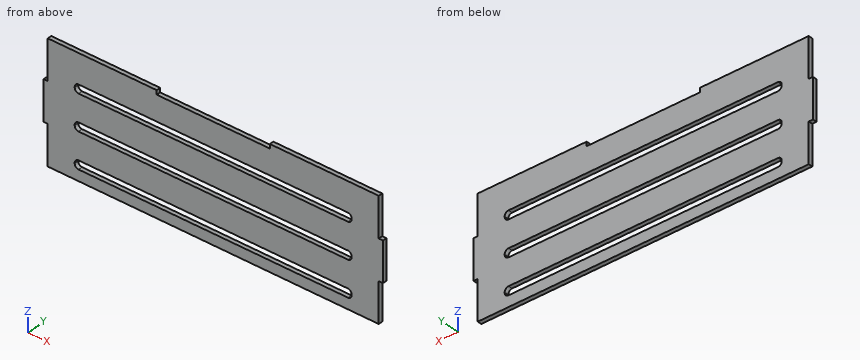
from build123d import *

# Parameters (mm, degrees)
SKETCH1_W           = 490
SKETCH1_H           = 168.89
BOSS_EXTRUDE1_DEPTH = 6
SKETCH2_W           = 163.333333334
SKETCH2_H           = 6
CUT_EXTRUDE1_DEPTH  = 519.324060892
SKETCH4_W           = 6
SKETCH4_H           = 56.296666667
CUT_EXTRUDE3_DEPTH  = 519.324060892
CUT_EXTRUDE4_DEPTH  = 519.324060892
LPATTERN1_COUNT     = 3
LPATTERN1_PITCH     = 50


with BuildPart() as part:
    # Sketch1 → Boss-Extrude1 (new body)
    with BuildSketch(Plane(origin=(0, 0, 0), x_dir=(1, 0, 0), z_dir=(0, 1, 0))):
        with Locations((245, 84.445)):
            Rectangle(SKETCH1_W, SKETCH1_H)
    extrude(amount=BOSS_EXTRUDE1_DEPTH)

    # Sketch2 → Cut-Extrude1 (cut, through all)
    with BuildSketch(Plane(origin=(0, 6, 0), x_dir=(1, 0, 0), z_dir=(0, 1, 0))):
        with Locations((245, 3)):
            Rectangle(SKETCH2_W, SKETCH2_H)
    extrude(amount=-CUT_EXTRUDE1_DEPTH, mode=Mode.SUBTRACT)

    # Sketch4 → Cut-Extrude3 (cut, through all)
    with BuildSketch(Plane(origin=(0, 6, 0), x_dir=(1, 0, 0), z_dir=(0, 1, 0))):
        with Locations((3, 140.741666667)):
            Rectangle(SKETCH4_W, SKETCH4_H)
        with Locations((3, 28.148333334)):
            Rectangle(SKETCH4_W, SKETCH4_H)
        with Locations((487, 28.148333334)):
            Rectangle(SKETCH4_W, SKETCH4_H)
        with Locations((487, 140.741666667)):
            Rectangle(SKETCH4_W, SKETCH4_H)
    extrude(amount=-CUT_EXTRUDE3_DEPTH, mode=Mode.SUBTRACT)

    # Sketch5 → Cut-Extrude4 (cut, through all)
    with BuildSketch(Plane(origin=(0, 6, 0), x_dir=(1, 0, 0), z_dir=(0, 1, 0))):
        with BuildLine():
            Line((50.5, 153.449523313), (439.5, 153.449523313))
            ThreePointArc((439.5, 153.449523313), (443.389087297, 151.838610609), (445, 147.949523313))
            Line((445, 147.949523313), (445, 146.949523313))
            ThreePointArc((445, 146.949523313), (443.389087297, 143.060436016), (439.5, 141.449523313))
            Line((439.5, 141.449523313), (50.5, 141.449523313))
            ThreePointArc((50.5, 141.449523313), (46.610912703, 143.060436016), (45, 146.949523313))
            Line((45, 146.949523313), (45, 147.949523313))
            ThreePointArc((45, 147.949523313), (46.610912703, 151.838610609), (50.5, 153.449523313))
        make_face()
    cut_extrude4 = extrude(amount=-CUT_EXTRUDE4_DEPTH, mode=Mode.SUBTRACT)

    # LPattern1: Cut-Extrude4 ×3
    with Locations(*[(0, 0, i * LPATTERN1_PITCH) for i in range(1, LPATTERN1_COUNT)]):
        add(cut_extrude4, mode=Mode.SUBTRACT)


solid = part.part
Build history of the part. All positions in model axes, mm. Round coordinates to 2 decimals unless told otherwise and drop trailing zeros. Write each loop counter-clockwise with the first axis right and the second up, starting at its lowest first coordinate (ties: lowest second). Pieces come first, ordered by that corner, then holes. Notation, with made-up numbers: M 82,86.5 L 129,86.5 A31 ccw 129,123.5 Z; hole C -8.5,-26 d9. An arc over 180 degrees is marked long. Answer as a JSON object with one key per item and string values. Group by question number.
(1) Cut at D-D (z = -28). Give the cut face in (x, y), and give its area (3 significant figures).
(2) Cut at C-C (y = 2.3). Give the number of separate pieces and of enclosed holes in the cut face, and give its area (3 significant figures).
(3) Cut at A-A (x = 186). Give the cut face in (y, z), and give its area (3 significant figures).
(4) Flat gauge pins, fed straight in: pin 1 (1.1 mm diameter, centred on y = 2, z = -47.5, fed in from +X); pin 2 (1 mm diameter, centred on y = 4, z = -22, fed in from -X); pin 3 (1.8 mm diameter, centred on x = 311, y = 4, fed in from +Z). Where does each tip first touch, or does it go through?
(5) Cut at B-B (x = 373). Give the cut face in (y, z).
(6) Drill centre lines: L1, parallel to Z at x = 190, y = 4.9; L2, parallel to Z at x = 337, y = 3.4; L3, parallel to X at y = 1.05, z = -24.5. Where is each one in solid material? Low to high.
Responses:
{
 "1": {"outline": "M 6,0 L 484,0 L 484,6 L 6,6 Z", "area": "2,870 mm2"},
 "2": {"separate pieces": "1", "enclosed holes": "3", "area": "66,100 mm2"},
 "3": {"outline": "M 0,-168.89 L 6,-168.89 L 6,-153.45 L 0,-153.45 Z; M 0,-141.45 L 6,-141.45 L 6,-103.45 L 0,-103.45 Z; M 0,-91.45 L 6,-91.45 L 6,-53.45 L 0,-53.45 Z; M 0,-41.45 L 6,-41.45 L 6,-6 L 0,-6 Z", "area": "761 mm2"},
 "4": {"pin 1": "stops at x = 484", "pin 2": "stops at x = 6", "pin 3": "stops at z = -6"},
 "5": {"outline": "M 0,-168.89 L 6,-168.89 L 6,-153.45 L 0,-153.45 Z; M 0,-141.45 L 6,-141.45 L 6,-103.45 L 0,-103.45 Z; M 0,-91.45 L 6,-91.45 L 6,-53.45 L 0,-53.45 Z; M 0,-41.45 L 6,-41.45 L 6,0 L 0,0 Z"},
 "6": {"L1": "z = -168.89 to -153.45, -141.45 to -103.45, -91.45 to -53.45, -41.45 to -6", "L2": "z = -168.89 to -153.45, -141.45 to -103.45, -91.45 to -53.45, -41.45 to 0", "L3": "x = 6 to 484"}
}
